Geometry check sheet. Reference: the model listing, model coordinates, mm. Face numbers are marked on the shaded views. A direction names the side the tool comes from. Round coordinates to 2 decimals unless told otherwise and drop trailing zeros. Order: outer loops, then holes, each group sorted by start corner. A loop starts at its lowest first (then second) coordinate and runs counter-clockwise, first axis right, second up.
(1) Release check for a two-part mould opening along Y. For the marked faces 1, 2 and 3 record: +Y half, -Y half, draft (parallel to the pull), parting line (faces both ways), or undercut.
(2) Sectioned sample at A-A (z = 5). Record the boundary of the cut face in (x, y).
(3) Set-up check for the marked faces 4, 5, 6 and 7: record each of +Z, -Z, +X, -X, +Y, -Y from which the full face is reachable in a straight line by a thin tool's end or side.
(4) Sectioned sample at D-D (z = 11.25). Record the boundary of the cut face in (x, y).
(5) Sectioned sample at B-B (y = -22). Record the boundary of the cut face in (x, z).
(6) Sectioned sample at C-C (y = 0). Record the boundary of the cut face in (x, z), plus the area to 3 significant figures.
(7) Go/stop test with flat-tipped pins: pin 1 (0.6 mm diameter, centred on x = 8.5, z = 11, fed in from +Y); pin 2 (4.5 mm diameter, centred on x = 17, y = 0, fed in from -Z); pin 3 (1.6 mm diameter, centred on x = 18, z = 9.5, fed in from +Y). Record where each tip stops, or that it passes through.
(8) Material ranges on line 1 along X through (y, z) = (0, 1.4); line 2 along Z through (x, y) = (12, 10); line 3 along Z through (x, y) = (0.75, 22), recorded low to high.
from build123d import *

# Parameters (mm, degrees)
F0_W      = 15
F0_H      = 2
F0_R      = 1.75
F1_DEPTH  = 2
F2_DEPTH  = 2
F3_DEPTH  = 2.5
F4_W      = 6
F4_H      = 26
F5_DEPTH  = 7
F6_DEPTH  = 6
F7_R      = 1.75
F8_DEPTH  = 2
F9_DEPTH  = 0.5
F10_W     = 9
F10_H     = 2
F11_DEPTH = 2
F12_R     = 2
F13_DEPTH = 25
F14_R     = 1.75
F15_DEPTH = 1
F16_W     = 6
F16_H     = 1
F17_DEPTH = 15


with BuildPart() as f1:
    # F0 (on Top) → F1 (new body)
    with BuildSketch(Plane.XY):
        with BuildLine():
            Line((15, -9.5), (0, -9.5))
            Line((0, -9.5), (0, -30))
            Line((0, -30), (2, -30))
            Line((2, -30), (2, -18.25))
            Line((2, -18.25), (7.7660733269, -18.25))
            Line((7.7660733269, -18.25), (7.7660733269, -15.5))
            ThreePointArc((7.7660733269, -15.5), (9.1573161163, -12.1412427894), (12.5160733269, -10.75))
            Line((12.5160733269, -10.75), (15, -10.75))
            Line((15, -10.75), (15, -9.5))
        make_face()
        with BuildLine():
            Line((0, 30), (0, 9.5))
            Line((0, 9.5), (15, 9.5))
            Line((15, 9.5), (15, 10.75))
            Line((15, 10.75), (12.5160733269, 10.75))
            ThreePointArc((12.5160733269, 10.75), (9.1573161163, 12.1412427894), (7.7660733269, 15.5))
            Line((7.7660733269, 15.5), (7.7660733269, 18.25))
            Line((7.7660733269, 18.25), (2, 18.25))
            Line((2, 18.25), (2, 30))
            Line((2, 30), (0, 30))
        make_face()
        Polygon((19.5, -5.8877859777), (19.5, -4.617), (19.5, -4.5), (0, -4.5), (0, -7.5), (15, -7.5), (15, -7), (15, -6), (19.5, -6), align=None)
        with BuildLine():
            Line((18.1456439237, -2.5), (19.5, -2.5))
            Line((19.5, -2.5), (19.5, -1.1456439237))
            ThreePointArc((19.5, -1.1456439237), (18.9445436483, -1.9445436483), (18.1456439237, -2.5))
        make_face()
        with Locations((7.5, -8.5)):
            Rectangle(F0_W, F0_H)
        with Locations((7.5, 8.5)):
            Rectangle(F0_W, F0_H)
        Polygon((0, 7.5), (0, 4.5), (19.5, 4.5), (19.5, 4.617), (19.5, 5.8877859777), (19.5, 6), (15, 6), (15, 7), (15, 7.5), align=None)
        with BuildLine():
            ThreePointArc((18.1456439237, 2.5), (18.9445436483, 1.9445436483), (19.5, 1.1456439237))
            Line((19.5, 1.1456439237), (19.5, 2.5))
            Line((19.5, 2.5), (18.1456439237, 2.5))
        make_face()
        with BuildLine():
            Line((0, 0), (0, -2.5))
            Line((0, -2.5), (15.8543560763, -2.5))
            ThreePointArc((15.8543560763, -2.5), (14.25, 0), (15.8543560763, 2.5))
            Line((15.8543560763, 2.5), (0, 2.5))
            Line((0, 2.5), (0, 0))
        make_face()
        with BuildLine():
            Line((0, -4.5), (19.5, -4.5))
            Line((19.5, -4.5), (19.5, -2.5))
            Line((19.5, -2.5), (18.1456439237, -2.5))
            ThreePointArc((18.1456439237, -2.5), (17, -2.75), (15.8543560763, -2.5))
            Line((15.8543560763, -2.5), (0, -2.5))
            Line((0, -2.5), (0, -4.5))
        make_face()
        with BuildLine():
            Line((0, 2.5), (15.8543560763, 2.5))
            ThreePointArc((15.8543560763, 2.5), (17, 2.75), (18.1456439237, 2.5))
            Line((18.1456439237, 2.5), (19.5, 2.5))
            Line((19.5, 2.5), (19.5, 4.5))
            Line((19.5, 4.5), (0, 4.5))
            Line((0, 4.5), (0, 2.5))
        make_face()
        with BuildLine():
            ThreePointArc((18.1456439237, -2.5), (18.9445436483, -1.9445436483), (19.5, -1.1456439237))
            Line((19.5, -1.1456439237), (19.5, 0.8877859777))
            Line((19.5, 0.8877859777), (19.5, 1.1456439237))
            ThreePointArc((19.5, 1.1456439237), (18.9445436483, 1.9445436483), (18.1456439237, 2.5))
            Line((18.1456439237, 2.5), (15.8543560763, 2.5))
            ThreePointArc((15.8543560763, 2.5), (14.25, 0), (15.8543560763, -2.5))
            Line((15.8543560763, -2.5), (18.1456439237, -2.5))
        make_face()
        with Locations((17, 0)):
            Circle(F0_R, mode=Mode.SUBTRACT)
    extrude(amount=F1_DEPTH)

    # F0 (on Top) → F2 (join)
    with BuildSketch(Plane.XY):
        with Locations((7.5, -8.5)):
            Rectangle(F0_W, F0_H)
        with BuildLine():
            Line((0, -4.5), (19.5, -4.5))
            Line((19.5, -4.5), (19.5, -2.5))
            Line((19.5, -2.5), (18.1456439237, -2.5))
            ThreePointArc((18.1456439237, -2.5), (17, -2.75), (15.8543560763, -2.5))
            Line((15.8543560763, -2.5), (0, -2.5))
            Line((0, -2.5), (0, -4.5))
        make_face()
        with BuildLine():
            Line((0, 2.5), (15.8543560763, 2.5))
            ThreePointArc((15.8543560763, 2.5), (17, 2.75), (18.1456439237, 2.5))
            Line((18.1456439237, 2.5), (19.5, 2.5))
            Line((19.5, 2.5), (19.5, 4.5))
            Line((19.5, 4.5), (0, 4.5))
            Line((0, 4.5), (0, 2.5))
        make_face()
        with Locations((7.5, 8.5)):
            Rectangle(F0_W, F0_H)
    extrude(amount=-F2_DEPTH)

    # F0 (on Top) → F3 (join)
    with BuildSketch(Plane.XY):
        with BuildLine():
            ThreePointArc((18.1456439237, -2.5), (18.9445436483, -1.9445436483), (19.5, -1.1456439237))
            Line((19.5, -1.1456439237), (19.5, 0.8877859777))
            Line((19.5, 0.8877859777), (19.5, 1.1456439237))
            ThreePointArc((19.5, 1.1456439237), (18.9445436483, 1.9445436483), (18.1456439237, 2.5))
            Line((18.1456439237, 2.5), (15.8543560763, 2.5))
            ThreePointArc((15.8543560763, 2.5), (14.25, 0), (15.8543560763, -2.5))
            Line((15.8543560763, -2.5), (18.1456439237, -2.5))
        make_face()
        with Locations((17, 0)):
            Circle(F0_R, mode=Mode.SUBTRACT)
        with BuildLine():
            ThreePointArc((15.8543560763, -2.5), (17, -2.75), (18.1456439237, -2.5))
            Line((18.1456439237, -2.5), (15.8543560763, -2.5))
        make_face()
        with BuildLine():
            ThreePointArc((18.1456439237, 2.5), (17, 2.75), (15.8543560763, 2.5))
            Line((15.8543560763, 2.5), (18.1456439237, 2.5))
        make_face()
    extrude(amount=F3_DEPTH)

    # F4 (on face) → F5 (cut)
    with BuildSketch(Plane.XY.offset(2)):
        with Locations((3, 0)):
            Rectangle(F4_W, F4_H)
    extrude(amount=-F5_DEPTH, mode=Mode.SUBTRACT)

    # F4 (on face) → F6 (join)
    with BuildSketch(Plane.XY.offset(2)):
        with BuildLine():
            Line((8, -7.5), (8, -4.5))
            Line((8, -4.5), (8, -2.5))
            Line((8, -2.5), (8, 2.5))
            Line((8, 2.5), (8, 4.5))
            Line((8, 4.5), (8, 7.5))
            Line((8, 7.5), (8, 9.5))
            Line((8, 9.5), (8, 14.0277290651))
            ThreePointArc((8, 14.0277290651), (7.8249195082, 14.7546303947), (7.7660733269, 15.5))
            Line((7.7660733269, 15.5), (7.7660733269, 18.25))
            Line((7.7660733269, 18.25), (2, 18.25))
            Line((2, 18.25), (2, 30))
            Line((2, 30), (0, 30))
            Line((0, 30), (0, 13))
            Line((0, 13), (6, 13))
            Line((6, 13), (6, -13))
            Line((6, -13), (0, -13))
            Line((0, -13), (0, -30))
            Line((0, -30), (2, -30))
            Line((2, -30), (2, -18.25))
            Line((2, -18.25), (7.7660733269, -18.25))
            Line((7.7660733269, -18.25), (7.7660733269, -15.5))
            ThreePointArc((7.7660733269, -15.5), (7.8249195082, -14.7546303947), (8, -14.0277290651))
            Line((8, -14.0277290651), (8, -9.5))
            Line((8, -9.5), (8, -7.5))
        make_face()
    extrude(amount=F6_DEPTH)

    # F7 (on face) → F8 (join)
    with BuildSketch(Plane.XY.offset(8)):
        with BuildLine():
            ThreePointArc((7.7660733269, -15.5), (7.8249195082, -14.7546303947), (8, -14.0277290651))
            Line((8, -14.0277290651), (8, 14.0277290651))
            ThreePointArc((8, 14.0277290651), (7.8249195082, 14.7546303947), (7.7660733269, 15.5))
            Line((7.7660733269, 15.5), (7.7660733269, 18.25))
            Line((7.7660733269, 18.25), (2, 18.25))
            Line((2, 18.25), (2, 30))
            Line((2, 30), (0, 30))
            Line((0, 30), (0, 13))
            Line((0, 13), (6, 13))
            Line((6, 13), (6, -13))
            Line((6, -13), (0, -13))
            Line((0, -13), (0, -30))
            Line((0, -30), (2, -30))
            Line((2, -30), (2, -18.25))
            Line((2, -18.25), (7.7660733269, -18.25))
            Line((7.7660733269, -18.25), (7.7660733269, -15.5))
        make_face()
        with BuildLine():
            Line((19.5, -5.8877859777), (19.5, -4.617))
            Line((19.5, -4.617), (19.5, -1.1456439237))
            ThreePointArc((19.5, -1.1456439237), (14.25, 0), (19.5, 1.1456439237))
            Line((19.5, 1.1456439237), (19.5, 4.617))
            Line((19.5, 4.617), (19.5, 5.8877859777))
            Line((19.5, 5.8877859777), (19.5, 6))
            Line((19.5, 6), (15, 6))
            Line((15, 6), (15, 7))
            Line((15, 7), (15, 10.75))
            Line((15, 10.75), (12.5160733269, 10.75))
            ThreePointArc((12.5160733269, 10.75), (9.7259825525, 11.6557974207), (8, 14.0277290651))
            Line((8, 14.0277290651), (8, -14.0277290651))
            ThreePointArc((8, -14.0277290651), (9.7259825525, -11.6557974207), (12.5160733269, -10.75))
            Line((12.5160733269, -10.75), (15, -10.75))
            Line((15, -10.75), (15, -7))
            Line((15, -7), (15, -6))
            Line((15, -6), (19.5, -6))
            Line((19.5, -6), (19.5, -5.8877859777))
        make_face()
        with BuildLine():
            ThreePointArc((19.5, 1.1456439237), (14.25, 0), (19.5, -1.1456439237))
            Line((19.5, -1.1456439237), (19.5, 0.8877859777))
            Line((19.5, 0.8877859777), (19.5, 1.1456439237))
        make_face()
        with Locations((17, 0)):
            Circle(F7_R, mode=Mode.SUBTRACT)
    extrude(amount=F8_DEPTH)

    # F7 (on face) → F9 (join)
    with BuildSketch(Plane.XY.offset(8)):
        with BuildLine():
            ThreePointArc((19.5, 1.1456439237), (14.25, 0), (19.5, -1.1456439237))
            Line((19.5, -1.1456439237), (19.5, 0.8877859777))
            Line((19.5, 0.8877859777), (19.5, 1.1456439237))
        make_face()
        with Locations((17, 0)):
            Circle(F7_R, mode=Mode.SUBTRACT)
    extrude(amount=-F9_DEPTH)

    # F10 (on face) → F11 (join)
    with BuildSketch(Plane.XY.offset(10)):
        with Locations((10.5, 8.5)):
            Rectangle(F10_W, F10_H)
        Polygon((6, 4.5), (6, 2.5), (15.2679491924, 2.5), (15.4122867597, 2.75), (18.5877132403, 2.75), (18.7320508076, 2.5), (19.5, 2.5), (19.5, 4.5), align=None)
        Polygon((6, -4.5), (19.5, -4.5), (19.5, -2.5), (18.7320508076, -2.5), (18.5877132403, -2.75), (15.4122867597, -2.75), (15.2679491924, -2.5), (6, -2.5), align=None)
        with Locations((10.5, -8.5)):
            Rectangle(F10_W, F10_H)
    extrude(amount=F11_DEPTH)

    # F12 (on face) → F13 (cut)
    with BuildSketch(Plane(origin=(0, 0, 0), x_dir=(0, -1, 0), z_dir=(-1, 0, 0))):
        with Locations((-22, 5)):
            Circle(F12_R)
        with Locations((22, 5)):
            Circle(F12_R)
    extrude(amount=-F13_DEPTH, mode=Mode.SUBTRACT)

    # F14 (on face) → F15 (cut)
    with BuildSketch(Plane(origin=(0, 0, 0), x_dir=(1, 0, 0), z_dir=(0, 0, -1))):
        with BuildLine():
            ThreePointArc((19.5, 1.1456439237), (18.9445436483, 1.9445436483), (18.1456439237, 2.5))
            ThreePointArc((18.1456439237, 2.5), (17, 2.75), (15.8543560763, 2.5))
            ThreePointArc((15.8543560763, 2.5), (14.25, 0), (15.8543560763, -2.5))
            ThreePointArc((15.8543560763, -2.5), (17, -2.75), (18.1456439237, -2.5))
            ThreePointArc((18.1456439237, -2.5), (18.9445436483, -1.9445436483), (19.5, -1.1456439237))
            Line((19.5, -1.1456439237), (19.5, 1.1456439237))
        make_face()
        with Locations((17, 0)):
            Circle(F14_R, mode=Mode.SUBTRACT)
    extrude(amount=-F15_DEPTH, mode=Mode.SUBTRACT)

    # F16 (on face) → F17 (cut, symmetric)
    with BuildSketch(Plane.XY.offset(8)):
        with Locations((3, -13.5)):
            Rectangle(F16_W, F16_H)
        with Locations((3, 13.5)):
            Rectangle(F16_W, F16_H)
    extrude(amount=F17_DEPTH, both=True, mode=Mode.SUBTRACT)


solid = f1.part
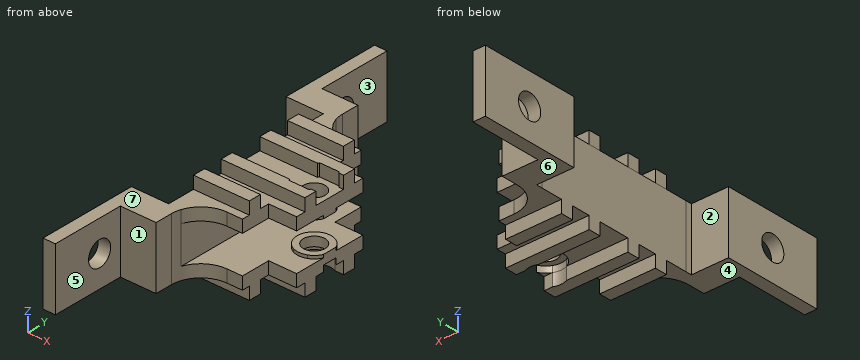
Answer below:
1. face 1: -Y half
1. face 2: undercut
1. face 3: draft
2. outline: (0, -30) - (2, -30) - (2, -24) - (0, -24) - close; (0, -20) - (2, -20) - (2, -18.25) - (7.77, -18.25) - (7.77, -15.5) arc R4.75 cw to (8, -14.03) - (8, 14.03) arc R4.75 cw to (7.77, 15.5) - (7.77, 18.25) - (2, 18.25) - (2, 20) - (0, 20) - (0, 14) - (6, 14) - (6, -14) - (0, -14) - close; (0, 24) - (2, 24) - (2, 30) - (0, 30) - close
3. face 4: -Z, +X, -X, -Y
3. face 5: +Z, -Z, +X, -Y
3. face 6: -Z, +X, -X, +Y
3. face 7: +Z, +X, -X, -Y
4. outline: (6, -9.5) - (15, -9.5) - (15, -7.5) - (6, -7.5) - close; (6, -4.5) - (19.5, -4.5) - (19.5, -2.5) - (18.73, -2.5) - (18.59, -2.75) - (15.41, -2.75) - (15.27, -2.5) - (6, -2.5) - close; (6, 2.5) - (15.27, 2.5) - (15.41, 2.75) - (18.59, 2.75) - (18.73, 2.5) - (19.5, 2.5) - (19.5, 4.5) - (6, 4.5) - close; (6, 7.5) - (15, 7.5) - (15, 9.5) - (6, 9.5) - close
5. outline: (0, 0) - (2, 0) - (2, 3) - (0, 3) - close; (0, 7) - (2, 7) - (2, 10) - (0, 10) - close
6. outline: (6, 0) - (14.25, 0) - (14.25, 1) - (15.25, 1) - (15.25, 2.5) - (14.25, 2.5) - (14.25, 2) - (8, 2) - (8, 8) - (14.25, 8) - (14.25, 7.5) - (15.25, 7.5) - (15.25, 10) - (6, 10) - close; (18.75, 1) - (19.5, 1) - (19.5, 2.5) - (18.75, 2.5) - close; (18.75, 7.5) - (19.5, 7.5) - (19.5, 10) - (18.75, 10) - close
6. area: 52.0 mm2
7. pin 1: stops at y = 9.5
7. pin 2: stops at z = 1
7. pin 3: stops at y = 6
8. line 1: x = 6 to 15.25, 18.75 to 19.5
8. line 2: z = 0 to 2, 8 to 10
8. line 3: z = 0 to 3, 7 to 10
